Part model, mm, in its own coordinate system. Coordinates: 2 decimals unless noted, no trailing zeros. Loops run counter-clockwise (first coordinate to the right, second up) from the corner with the lowest first, then second, coordinate; pieces in that order, holes last. Notation, with made-up numbers: (15.5, 82.5) - (39.5, 82.5) arc R32 cw to (39.5, 109.5) - close; hole circle Ø11 at (-25.5, 30.5). An arc over 180 degrees is marked (long way). Use a Markdown table: item, result. Add a question column.
1) Probe probe 1 along X at (y, z) = (-0.5, -11.5); probe 2 along X at (y, z) = (-1.5, 17); probe 3 along X at (y, z) = (-0.5, -20). List the from-to ranges inside material, lowest first. Write a range as [from, to].
2) Band-saw the part on A-A (z = 4.5). Give the cut face in (x, y) (3 decimals).
3) Band-saw the part on B-B (y = -2.05). Give the cut face in (x, z) (1 decimal), plus the area to 3 significant figures.
4) Band-saw the part on D-D (x = -52.5). Give the cut face in (y, z) (3 decimals), plus the area to 3 significant figures.
5) Band-saw the part on C-C (z = 15.5). Give the cut face in (x, y) (3 decimals).
6) Drop flat-ended pins along their axis: P1, Ø4, axis at x = -63.5, z = 4, coming from the +Y side; P2, Ø1.6, axis at x = -48, y = -1, coming from the -Z side; P3, Ø1, axis at x = -51.5, y = -2, coming from the -Z side. Give the stop position or say it passes through.
from build123d import *

# Parameters (mm, degrees)
F0_R     = 1.5875
F1_DEPTH = 3.175


with BuildPart() as f1:
    # F0 (on Front) → F1 (new body)
    with BuildSketch(Plane.XZ):
        with BuildLine():
            Line((-45.703146, 7.703695), (-45.703146, -49.446305))
            Line((-45.703146, -49.446305), (-26.653146, -49.446305))
            Line((-26.653146, -49.446305), (-26.653146, 16.593695))
            ThreePointArc((-26.653146, 16.593695), (-29.628941, 23.7779), (-36.813146, 26.753695))
            Line((-36.813146, 26.753695), (-45.703146, 26.753695))
            Line((-45.703146, 26.753695), (-107.68587, 26.753695))
            ThreePointArc((-107.68587, 26.753695), (-113.98265, 24.567161), (-117.56917, 18.948688))
            ThreePointArc((-117.56917, 18.948688), (-117.776458, 17.779291), (-117.84587, 16.593695))
            Line((-117.84587, 16.593695), (-117.84587, 7.703695))
            Line((-117.84587, 7.703695), (-117.84587, -49.446305))
            Line((-117.84587, -49.446305), (-98.79587, -49.446305))
            Line((-98.79587, -49.446305), (-98.79587, 7.703695))
            Line((-98.79587, 7.703695), (-53.83787, 7.703695))
            Line((-53.83787, 7.703695), (-53.83787, 17.863695))
            Line((-53.83787, 17.863695), (-50.66287, 17.863695))
            Line((-50.66287, 17.863695), (-50.66287, 7.703695))
            Line((-50.66287, 7.703695), (-45.703146, 7.703695))
        make_face()
        with Locations((-108.32087, -30.639023)):
            Circle(F0_R, mode=Mode.SUBTRACT)
        with Locations((-108.32087, -11.346305)):
            Circle(F0_R, mode=Mode.SUBTRACT)
        with Locations((-108.32087, 8.285769)):
            Circle(F0_R, mode=Mode.SUBTRACT)
    extrude(amount=F1_DEPTH)


solid = f1.part
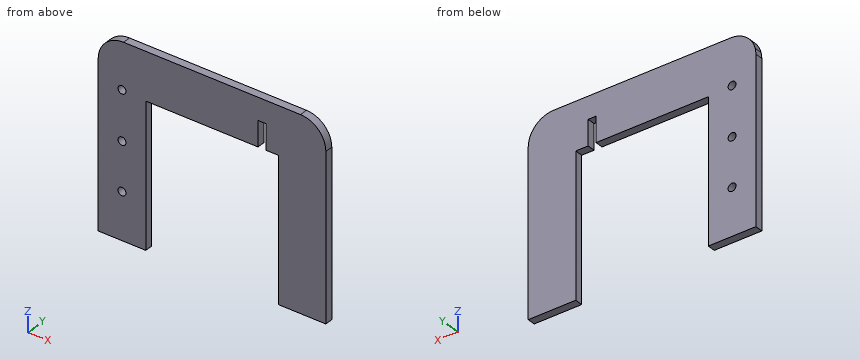
Answer block:
| question | item | result |
|---|---|---|
| 1 | probe 1 | [-117.85, -109.9], [-106.74, -98.8], [-45.7, -26.65] |
| 1 | probe 2 | [-117.84, -53.84], [-50.66, -26.66] |
| 1 | probe 3 | [-117.85, -98.8], [-45.7, -26.65] |
| 2 | outline | (-117.846, -3.175) - (-98.796, -3.175) - (-98.796, 0) - (-117.846, 0) - close; (-45.703, -3.175) - (-26.653, -3.175) - (-26.653, 0) - (-45.703, 0) - close |
| 3 | outline | (-117.8, -49.4) - (-98.8, -49.4) - (-98.8, 7.7) - (-53.8, 7.7) - (-53.8, 17.9) - (-50.7, 17.9) - (-50.7, 7.7) - (-45.7, 7.7) - (-45.7, -49.4) - (-26.7, -49.4) - (-26.7, 16.6) arc R10.2 ccw to (-36.8, 26.8) - (-107.7, 26.8) arc R10.2 ccw to (-117.6, 18.9) arc R10.2 ccw to (-117.8, 16.6) - close; hole circle Ø3.2 at (-108.3, -30.6); hole circle Ø3.2 at (-108.3, -11.3); hole circle Ø3.2 at (-108.3, 8.3) |
| 3 | area | 3,810 mm2 |
| 4 | outline | (-3.175, 17.864) - (0, 17.864) - (0, 26.754) - (-3.175, 26.754) - close |
| 4 | area | 28.2 mm2 |
| 5 | outline | (-117.846, -3.175) - (-53.838, -3.175) - (-53.838, 0) - (-117.846, 0) - close; (-50.663, -3.175) - (-26.653, -3.175) - (-26.653, 0) - (-50.663, 0) - close |
| 6 | P1 | through |
| 6 | P2 | z = 7.7 |
| 6 | P3 | z = 17.86 |
